Check sheet for the modelled part. Datum: model origin and axes. Units: mm. A direction names the side the tool comes from. Round coordinates to 2 decimals unless told otherwise and drop trailing zeros. Write each loop counter-clockwise with the first axis right and the second up, starting at its lowest first coordinate (ties: lowest second). Pieces come first, ordered by that corner, then holes.
Item 1: Cross-section at B-B on y = 1.85. Count the separate pieces of the cut face and the enclosed holes in it, plus the area to 3 significant figures.
Item 2: Material ranges on line 1 (X direction, y = 2.4, z = -30); line 2 (X direction, y = 2.3, z = -15); line 3 (X direction, y = 1.25, z = -32), recorded low to high.
Item 3: Cross-section at A-A on z = 25. Enter the section's corners in (x, y).
Item 4: Cross-section at D-D on x = -5. Enter the section's corners in (y, z).
Item 5: Cross-section at C-C on x = 0. Enter the section's corners in (y, z), plus the area to 3 significant figures.
Item 6: Tool access check on faces 1 (the flat face through (-25, 1, 1)), 2 (the cylindrical face through (-18.5, 1.5, 25.1)). Record the directions out of +Z, -Z, +X, -X, +Y, -Y that give a thin tool (end or side, any length) a straight path to the whole face; none if there is none.
Item 7: Release check for a two-part mould opening along Z. For faces 3 (the flat face through (0, 1, -40)), 4 (the cylindrical face through (-18.735, 1.521, 0.806)), 5 (the flat face through (25, 1, 1)) record: +Z half, -Z half, draft (parallel to the pull), parting line (faces both ways), or undercut.
from build123d import *

# Parameters (mm, degrees)
SKETCH1_W           = 50
SKETCH1_H           = 80
SKETCH1_R           = 2.5
SKETCH1_R_2         = 14
BOSS_EXTRUDE1_DEPTH = 3
SKETCH2_R           = 1.5
CUT_EXTRUDE1_DEPTH  = 10


with BuildPart() as part:
    # Sketch1 → Boss-Extrude1 (new body)
    with BuildSketch(Plane(origin=(0, 0, 0), x_dir=(1, 0, 0), z_dir=(0, 1, 0))):
        Rectangle(SKETCH1_W, SKETCH1_H)
        with Locations(Location((0, 32, 0), (0, 0, 270))):
            Circle(SKETCH1_R, mode=Mode.SUBTRACT)
        with Locations(Location((17, 15, 0), (0, 0, 270))):
            Circle(SKETCH1_R, mode=Mode.SUBTRACT)
        with Locations(Location((0, -2, 0), (0, 0, 270))):
            Circle(SKETCH1_R, mode=Mode.SUBTRACT)
        with Locations(Location((-17, 15, 0), (0, 0, 270))):
            Circle(SKETCH1_R, mode=Mode.SUBTRACT)
        with Locations(Location((0, 15, 0), (0, 0, 270))):
            Circle(SKETCH1_R_2, mode=Mode.SUBTRACT)
        with BuildLine():
            Line((-15, -21.5), (15, -21.5))
            ThreePointArc((15, -21.5), (18.5, -25), (15, -28.5))
            Line((15, -28.5), (-15, -28.5))
            ThreePointArc((-15, -28.5), (-18.5, -25), (-15, -21.5))
        make_face(mode=Mode.SUBTRACT)
    extrude(amount=BOSS_EXTRUDE1_DEPTH)

    # Sketch2 → Cut-Extrude1 (cut)
    with BuildSketch(Plane(origin=(0, 3, 0), x_dir=(1, 0, 0), z_dir=(0, 1, 0))):
        with Locations(Location((-20, 30, 0), (0, 0, 270))):
            Circle(SKETCH2_R)
        with Locations(Location((-20, 0, 0), (0, 0, 270))):
            Circle(SKETCH2_R)
    extrude(amount=-CUT_EXTRUDE1_DEPTH, mode=Mode.SUBTRACT)


solid = part.part
Response values:
1. separate pieces: 1
1. enclosed holes: 8
1. area: 3,040 mm2
2. line 1: x = -25 to -21.5, -18.5 to -1.5, 1.5 to 25
2. line 2: x = -25 to -19.5, -14.5 to -14, 14 to 14.5, 19.5 to 25
2. line 3: x = -25 to -2.5, 2.5 to 25
3. outline: (-25, 0) - (-18.5, 0) - (-18.5, 3) - (-25, 3) - close; (18.5, 0) - (25, 0) - (25, 3) - (18.5, 3) - close
4. outline: (0, -40) - (3, -40) - (3, -28.08) - (0, -28.08) - close; (0, -1.92) - (3, -1.92) - (3, 21.5) - (0, 21.5) - close; (0, 28.5) - (3, 28.5) - (3, 40) - (0, 40) - close
5. outline: (0, -40) - (3, -40) - (3, -34.5) - (0, -34.5) - close; (0, -29.5) - (3, -29.5) - (3, -29) - (0, -29) - close; (0, -1) - (3, -1) - (3, -0.5) - (0, -0.5) - close; (0, 4.5) - (3, 4.5) - (3, 21.5) - (0, 21.5) - close; (0, 28.5) - (3, 28.5) - (3, 40) - (0, 40) - close
5. area: 105 mm2
6. face 1: +Z, -Z, -X, +Y, -Y
6. face 2: +Y, -Y
7. face 3: -Z half
7. face 4: undercut
7. face 5: draft
